Could you check a few things on this model? Use its own coordinates, in mm. Face numbers are marked on the shaded views. A direction names the side the tool comes from. Coordinates: 2 decimals unless noted, no trailing zeros. Order: outer loops, then holes, each group sorted by start corner. A loop starts at its lowest first (then second) coordinate and runs counter-clockwise, first axis right, second up. Notation, with made-up numbers: M 88.25,5 L 134.25,5 A30 ccw 134.25,35 Z; hole C -18,-7 d4. An arc over 180 degrees is marked long. One line per question, with ' | ' between items. Start each with the question number.
from build123d import *
from build123d.topology import SkipClean

# Parameters (mm, degrees)
BOSS_EXTRUDE1_DEPTH = 40
FILLET1_R           = 25
SKETCH3_R           = 60
SKETCH3_W           = 140
SKETCH3_H           = 240
CUT_EXTRUDE1_DEPTH  = 360.436212163
BOSS_EXTRUDE2_START = 50
BOSS_EXTRUDE2_DEPTH = 50


with BuildPart() as part:
    # Sketch2 → Boss-Extrude1 (new body)
    with BuildSketch(Plane.XZ.offset(-202.963495408)):
        with BuildLine():
            Line((-139.764705882, 258.904671879), (-191.764705882, 161.404671879))
            ThreePointArc((-191.764705882, 161.404671879), (-197.90997501, 145.440989161), (-200, 128.463495408))
            Line((-200, 128.463495408), (-200, -129.036504592))
            ThreePointArc((-200, -129.036504592), (-178.033008589, -182.06951318), (-125, -204.036504592))
            Line((-125, -204.036504592), (125, -204.036504592))
            ThreePointArc((125, -204.036504592), (178.033008589, -182.06951318), (200, -129.036504592))
            Line((200, -129.036504592), (200, 128.463495408))
            ThreePointArc((200, 128.463495408), (197.90997501, 145.440989161), (191.764705882, 161.404671879))
            Line((191.764705882, 161.404671879), (139.764705882, 258.904671879))
            ThreePointArc((139.764705882, 258.904671879), (114.01470288, 285.988000208), (78, 295.963495408))
            Line((78, 295.963495408), (-78, 295.963495408))
            ThreePointArc((-78, 295.963495408), (-114.01470288, 285.988000208), (-139.764705882, 258.904671879))
        make_face()
    extrude(amount=BOSS_EXTRUDE1_DEPTH)

    # Fillet1
    fillet1_edges = [part.edges().sort_by_distance(p)[0] for p in [
        (-197.90997501, 162.963495408, 145.440989161),
        (-200, 162.963495408, -0.286504592),
        (-178.033008589, 162.963495408, -182.06951318),
        (0, 162.963495408, -204.036504592),
        (178.033008589, 162.963495408, -182.06951318),
        (200, 162.963495408, -0.286504592),
        (197.90997501, 162.963495408, 145.440989161),
        (165.764705882, 162.963495408, 210.154671879),
        (114.01470288, 162.963495408, 285.988000208),
        (0, 162.963495408, 295.963495408),
        (-114.01470288, 162.963495408, 285.988000208),
        (-165.764705882, 162.963495408, 210.154671879),
    ]]
    fillet(fillet1_edges, radius=FILLET1_R)

    # Sketch3 → Cut-Extrude1 (cut, through all)
    with BuildSketch(Plane.XZ.offset(-162.963495408)):
        with Locations(Location((0, 221, 0), (0, 0, 270))):
            Circle(SKETCH3_R)
        with Locations(Location((125, -129, 0), (0, 0, 270))):
            Circle(SKETCH3_R)
        with Locations(Location((-125, -129, 0), (0, 0, 270))):
            Circle(SKETCH3_R)
        with Locations((0, 25)):
            Rectangle(SKETCH3_W, SKETCH3_H)
    extrude(amount=-CUT_EXTRUDE1_DEPTH, mode=Mode.SUBTRACT)

    # Sketch4 → Boss-Extrude2 (add)
    with SkipClean():  # the faces are left unmerged after this step: merging them gives an invalid solid
        with BuildSketch(Plane.XZ.offset(-162.963495408).offset(BOSS_EXTRUDE2_START)):
            with BuildLine():
                Line((-70, 145), (-150, -20))
                Line((-150, -20), (-150, -69))
                Line((-150, -69), (-125, -69))
                ThreePointArc((-125, -69), (-82.573593129, -86.573593129), (-65, -129))
                Line((-65, -129), (-65, -175))
                Line((-65, -175), (65, -175))
                Line((65, -175), (65, -129))
                ThreePointArc((65, -129), (82.573593129, -86.573593129), (125, -69))
                Line((125, -69), (150, -69))
                Line((150, -69), (150, -20))
                Line((150, -20), (70, 145))
                Line((70, 145), (70, -95))
                Line((70, -95), (-70, -95))
                Line((-70, -95), (-70, 145))
            make_face()
        extrude(amount=-BOSS_EXTRUDE2_DEPTH)


solid = part.part
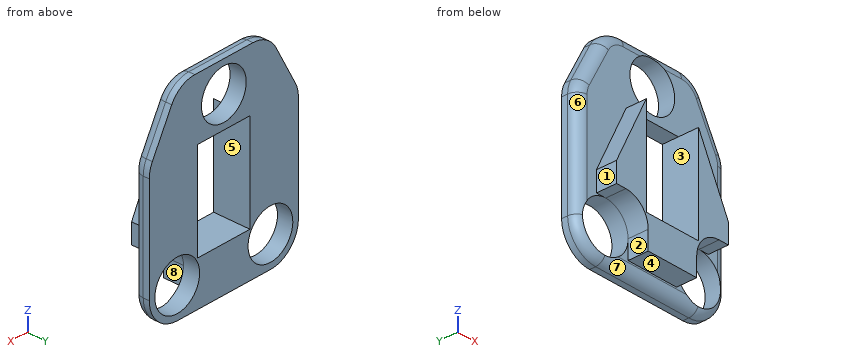
(1) Imagine slicing it at A-A, the plane y = 147.5. Write out the boundary of the cut face in (x, z).
(2) Imagine slicing it at C-C, the plane z = 16. Write out the boundary of the cut face in (x, y), plus the area to 3 significant figures.
(3) On a 3-axis mill with a long thin cutter (end or side, diameter ignored), from which of +Z, -Z, +X, -X, +Y, -Y can I reach the whole of each face in a straight line? I mean the marked faces 1, 2, 3 and 4. Say none if no direction works.
(4) Imagine slicing it at D-D, the plane y = 173. Write out the boundary of the cut face in (x, z).
(5) If I drill on line 1 along X through (y, z) = (191, -129); line 2 along Z through (x, y) = (0, 186); line 3 along X through (y, z) = (175, -129), over which ranges is the centre line in solid material (lowest first)? Write a range as from..to.
(6) We'd pull the mould along X, two halves only. Please class the marked faces 5, 6, 7 and 8: +X half, -X half, draft (parallel to the pull), parting line (faces both ways), or undercut.
(7) For P1, Ø1, axis at x = -51.5, y = 141, coming from the +Z side; P2, Ø12, axis at x = 5, y = 175.5, coming from the -Z side; P3, Ø2, axis at x = 56, y = 180.5, coming from the +Z side, each with a flat end and sliding along its axis, tell me the tip position at first contact or that it passes through.
(8) Imagine slicing it at B-B, the plane x = 0. Write out the boundary of the cut face in (y, z), plus the area to 3 significant figures.
Answers:
1) outline: M -150,-69 L -125,-69 A60 cw -65,-129 L -65,-175 L 65,-175 L 65,-129 A60 cw 125,-69 L 150,-69 L 150,-20 L 70,145 L 70,-95 L -70,-95 L -70,145 L -150,-20 Z
2) outline: M -200,187.96 A25 ccw -175,162.96 L -132.55,162.96 L -132.55,112.96 L -70,112.96 L -70,202.96 L -200,202.96 Z; M 70,112.96 L 132.55,112.96 L 132.55,162.96 L 175,162.96 A25 ccw 200,187.96 L 200,202.96 L 70,202.96 Z | area: 16,400 mm²
3) face 1: +Z, -Z, -X, -Y | face 2: -Z, -X, -Y | face 3: +Y, -Y | face 4: -Z, +X, -X, -Y
4) outline: M -195.03,-129.04 A70.03 ccw -125,-199.06 L 125,-199.06 A70.03 ccw 195.03,-129.04 L 195.03,128.46 A65.03 ccw 187.38,159.06 L 135.38,256.56 A65.03 ccw 78,290.99 L -78,290.99 A65.03 ccw -135.38,256.56 L -187.38,159.06 A65.03 ccw -195.03,128.46 Z; hole C -125,-129 d120; hole M -70,-95 L 70,-95 L 70,145 L -70,145 Z; hole C 0,221 d120; hole C 125,-129 d120
5) line 1: -200..-185, -65..65, 185..200 | line 2: -203.96..-95, 145..161, 281..295.89 | line 3: -196.38..-185, -65..65, 185..196.38
6) face 5: undercut | face 6: -X half | face 7: draft | face 8: +X half
7) P1: z = -95 | P2: z = -203.19 | P3: z = 295.11
8) outline: M 112.96,-175 L 162.96,-175 L 162.96,-179.04 A25 ccw 187.96,-204.04 L 202.96,-204.04 L 202.96,-95 L 112.96,-95 Z; M 162.96,145 L 202.96,145 L 202.96,161 L 162.96,161 Z; M 165.07,281 L 202.96,281 L 202.96,295.96 L 187.96,295.96 A25 ccw Z | area: 9,340 mm²
